```python
from build123d import *

# Parameters (mm, degrees)
SKETCH1_W           = 340
SKETCH1_H           = 340
BOSS_EXTRUDE1_DEPTH = 40
SKETCH2_R           = 50
CUT_EXTRUDE1_DEPTH  = 40


with BuildPart() as part:
    # Sketch1 → Boss-Extrude1 (new body)
    with BuildSketch(Plane(origin=(0, 0, 0), x_dir=(1, 0, 0), z_dir=(0, 1, 0))):
        Rectangle(SKETCH1_W, SKETCH1_H)
    extrude(amount=BOSS_EXTRUDE1_DEPTH)

    # Sketch2 → Cut-Extrude1 (cut)
    with BuildSketch(Plane(origin=(0, 40, 0), x_dir=(1, 0, 0), z_dir=(0, 1, 0))):
        Circle(SKETCH2_R)
    extrude(amount=-CUT_EXTRUDE1_DEPTH, mode=Mode.SUBTRACT)


solid = part.part
```
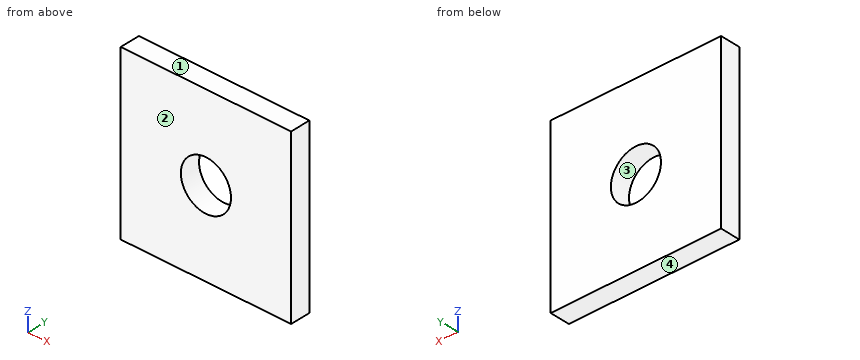
For this review, take the finished solid that the model builds, in its own axes (mm). Face numbers are marked on the shaded views. Coordinates: 2 decimals unless noted, no trailing zeros. Order: outer loops, then holes, each group sorted by start corner. A loop starts at its lowest first (then second) coordinate and runs counter-clockwise, first axis right, second up. Notation, with made-up numbers: (-12.75, 35.5) - (-7.75, 35.5) arc R13 ccw to (-7.75, 54.5) - close; hole circle Ø10 at (-26, 27). An arc over 180 degrees is marked (long way). Answer as a JSON object with one key per item and string values. Group by question number.
1. We need section A-A on z = 0. State the section outline as (x, y) points, then the cut area to 3 significant figures.
2. We need section C-C on y = 27.5. State the section outline as (x, z) points.
3. For probe 1 along X at (y, z) = (9, 0); probe 2 along Z at (x, y) = (18, 15.5), list the stretches that pass through material, from the lowest coordinate up.
4. We need section B-B on x = 0. State the section outline as (y, z) points, then the cut area to 3 significant figures.
5. The part is to be moulded in two halves that separate along Z. For the marked faces 1, 2, 3 and 4, say which applies: pulls with the +Z half, pulls with the -Z half, needs draft (parallel to the pull), parting line crosses it, or undercut.
Final values:
{
 "1": {"outline": "(-170, 0) - (-50, 0) - (-50, 40) - (-170, 40) - close; (50, 0) - (170, 0) - (170, 40) - (50, 40) - close", "area": "9,600 mm²"},
 "2": {"outline": "(-170, -170) - (170, -170) - (170, 170) - (-170, 170) - close; hole circle Ø100 at (0, 0)"},
 "3": {"probe 1": "-170 to -50, 50 to 170", "probe 2": "-170 to -46.65, 46.65 to 170"},
 "4": {"outline": "(0, -170) - (40, -170) - (40, -50) - (0, -50) - close; (0, 50) - (40, 50) - (40, 170) - (0, 170) - close", "area": "9,600 mm²"},
 "5": {"face 1": "pulls with the +Z half", "face 2": "needs draft", "face 3": "undercut", "face 4": "pulls with the -Z half"}
}
